Build history of the part. All positions in model axes, mm. Face numbers are marked on the shaded views. A direction names the side the tool comes from. Give positions to 0.01 mm unless a question says otherwise; leave off trailing zeros. Write each loop counter-clockwise with the first axis right and the second up, starting at its lowest first coordinate (ties: lowest second). Pieces come first, ordered by that corner, then holes. Notation, with made-up numbers: (72.5, 28) -> (110.5, 28) arc R20 ccw to (110.5, 58) -> close; hole circle Ø1 at (72, -27). An arc over 180 degrees is marked (long way). Put each result on its own line as item: value.
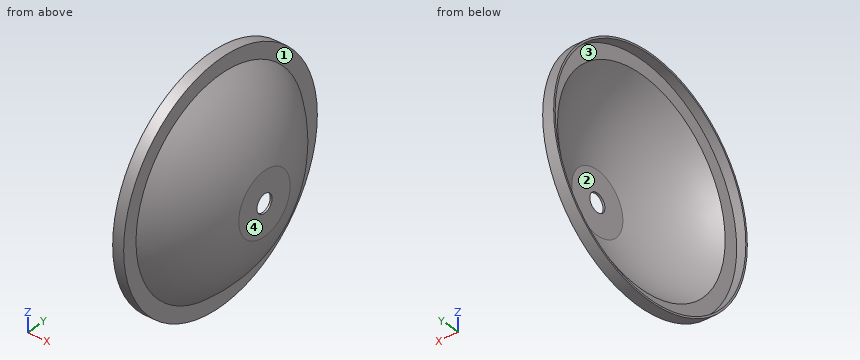
from build123d import *


with BuildPart() as part:
    # Sketch1 → Revolve1 (revolve)
    with BuildSketch(Plane.XY):
        with BuildLine():
            Line((41, 64), (47, 64))
            Line((47, 64), (47, 55.856960175))
            ThreePointArc((47, 55.856960175), (62.113205821, 38.352961589), (70.992957397, 17))
            Line((70.992957397, 17), (70.992957397, 5))
            Line((70.992957397, 5), (69.992957397, 5))
            Line((69.992957397, 5), (69.992957397, 16.881525843))
            ThreePointArc((69.992957397, 16.881525843), (61.108985686, 38.074819348), (46, 55.389529697))
            Line((46, 55.389529697), (46, 63))
            Line((46, 63), (41, 63))
            Line((41, 63), (41, 64))
        make_face()
    revolve(axis=Axis((0, 0, 0), (1, 0, 0)))


solid = part.part
1) Slice it at A-A (z = 0). Write the cut outline in (x, y), plus the area to 3 significant figures.
Filled sheet:
outline: (41, -64) -> (47, -64) -> (47, -55.86) arc R73 ccw to (70.99, -17) -> (70.99, -5) -> (69.99, -5) -> (69.99, -16.88) arc R72 cw to (46, -55.39) -> (46, -63) -> (41, -63) -> close; (41, 63) -> (46, 63) -> (46, 55.39) arc R72 cw to (69.99, 16.88) -> (69.99, 5) -> (70.99, 5) -> (70.99, 17) arc R73 ccw to (47, 55.86) -> (47, 64) -> (41, 64) -> close
area: 143 mm2
2) Pin check, flat tips, straight feed: pin 1 (1.5 mm diameter, centred on x = 59, y = 33, fed in from +Z); pin 2 (4 mm diameter, centred on x = 59, z = 16, fed in from +Y); pin 3 (10 mm diameter, centred on x = 55.5, y = -18, fed in from +Z). Stop position of each tip, or through.
Filled sheet:
pin 1: z = 29.32
pin 2: y = 42.81
pin 3: z = 49.83
3) Tool access for the marked faces 1 and 2: list every direction of +Z, -Z, +X, -X, +Y, -Y with a clear straight run to the whole face (end or side of a thin tool).
Filled sheet:
face 1: +X
face 2: -X
4) Slice it at D-D (z = -44.5). Write the cut outline in (x, y).
Filled sheet:
outline: (41, -46) -> (47, -46) -> (47, -33.76) arc R57.87 ccw to (47, 33.76) -> (47, 46) -> (41, 46) -> (41, 44.6) -> (46, 44.6) -> (46, 32.98) arc R56.6 cw to (46, -32.98) -> (46, -44.6) -> (41, -44.6) -> close
5) Pull direction Z, two halves, no side cores. Call the marked faces 3 and 4: released by +Z, released by -Z, zero draft, split by the parting line, or undercut.
Filled sheet:
face 3: undercut
face 4: zero draft
6) Slice it at C-C (y = -29). Write the cut outline in (x, z).
Filled sheet:
outline: (41, -57.05) -> (47, -57.05) -> (47, -47.74) arc R66.99 ccw to (47, 47.74) -> (47, 57.05) -> (41, 57.05) -> (41, 55.93) -> (46, 55.93) -> (46, 47.19) arc R65.9 cw to (46, -47.19) -> (46, -55.93) -> (41, -55.93) -> close
7) Wall check: L1, parallel to Z at x = 44.3, y = 0; L2, parallel to X at y = 43, z = -36.5; L3, parallel to X at y = -12.5, z = -2. Give the ranges that are in metal, low to high.
Filled sheet:
L1: -64 to -63, 63 to 64
L2: 46 to 47
L3: 69.99 to 70.99
